Source: CAD feature listing. Evaluate the final solid. Frame: model axes, mm. Face numbers are marked on the shaded views. A direction names the side the tool comes from. Round coordinates to 2 decimals unless told otherwise and drop trailing zeros. Loops run counter-clockwise (first coordinate to the right, second up) from the corner with the lowest first, then second, coordinate; pieces in that order, holes last. Notation, with made-up numbers: M 22,9.25 L 43,9.25 A20 cw 43,25.25 Z; hole C 13,1.25 d11. An arc over 180 degrees is marked long. Write each question's results on one line, items separated by ' | '. Start each with the question number.
1. Section D-D on z = 10. Output: boundary loops of the cut face in (x, y), and give its area (3 significant figures).
2. Draft query along Z for the marked faces 6, 7 and 8. Return one class per face: released by +Z, released by -Z, zero draft, split by the parting line, or undercut.
3. Contact query for flat-ended pins moving along their axis: pin 1 Ø8 at (y, z) = (45.5, 0.5) entering from -X; pin 2 Ø3 at (x, z) = (-0.5, -10.5) entering from +Y; pin 3 Ø12 at (x, z) = (-13, -4.5) entering from +Y. Output: stop coordinate, or through.
4. Section A-A on x = 0. Output: boundary loops of the cut face in (y, z) (3 decimals), and give its area (3 significant figures).
5. Section C-C on y = 52. Output: boundary loops of the cut face in (x, z).
6. Ray query, line 1 (X direction, y = 50, z = -6); line 2 (X direction, y = 32.5, z = 0.5); line 3 (Y direction, x = -9.5, z = -3). Return the intervals inside material, ascending.
7. Set-up query: the marked faces 1, 2, 3, 4 and 5. Return all of +Z, -Z, +X, -X, +Y, -Y with unobstructed straight access to the full face (end or side cutting, diameter ignored); none if empty.
8. Section B-B on z = 1. Output: boundary loops of the cut face in (x, y).
from build123d import *

# Parameters (mm, degrees)
SKETCH1_R               = 12.9921
BOSS_EXTRUDE1_DEPTH     = 25.4
CUT_EXTRUDE1_DEPTH      = 71.405666164
CUT_EXTRUDE1_DEPTH_BACK = 71.405666164
SKETCH3_R               = 3.81
CUT_REVOLVE1_ANGLE      = 270
CUT_REVOLVE2_ANGLE      = 270
SKETCH6_R               = 8.255
CUT_EXTRUDE2_DEPTH      = 2.032
CUT_EXTRUDE3_DEPTH      = 24.638


with BuildPart() as part:
    # Sketch1 → Boss-Extrude1 (new body)
    with BuildSketch(Plane(origin=(0, 0, 0), x_dir=(1, 0, 0), z_dir=(0, 1, 0))):
        with Locations(Location((0, 0, 0), (0, 0, 270))):
            Circle(SKETCH1_R)
    extrude(amount=BOSS_EXTRUDE1_DEPTH)

    # Sketch2 → Revolve1 (revolve)
    with BuildSketch(Plane(origin=(0, 0, 0), x_dir=(0, 0, -1), z_dir=(1, 0, 0))):
        with BuildLine():
            Line((-16.764, 25.4), (-16.764, 49.53))
            ThreePointArc((-16.764, 49.53), (-11.85393808, 61.38393808), (0, 66.294))
            Line((0, 66.294), (0, 25.4))
            Line((0, 25.4), (-16.764, 25.4))
        make_face()
    revolve(axis=Axis((0, 25.4, 0), (0, 1, 0)))

    # Sketch3 → Cut-Extrude1 (cut, two sides: drawn at the far end of the back side and taken through both)
    with BuildSketch(Plane(origin=(0, 0, 0), x_dir=(0, 0, -1), z_dir=(1, 0, 0)).offset(-CUT_EXTRUDE1_DEPTH_BACK)):
        with Locations((0, 49.53)):
            Circle(SKETCH3_R)
    extrude(amount=CUT_EXTRUDE1_DEPTH + CUT_EXTRUDE1_DEPTH_BACK, mode=Mode.SUBTRACT)

    # Sketch4 → Cut-Revolve1 (revolve, cut)
    with BuildSketch(Plane.XY):
        with BuildLine():
            Line((-7.62, 32.995439638), (-7.62, 49.53))
            Line((-7.62, 49.53), (7.62, 49.53))
            Line((7.62, 49.53), (7.62, 32.995439638))
            ThreePointArc((7.62, 32.995439638), (0, 31.32406453), (-7.62, 32.995439638))
        make_face()
    revolve(axis=Axis((-7.62, 49.53, 0), (1, 0, 0)), revolution_arc=CUT_REVOLVE1_ANGLE, mode=Mode.SUBTRACT)

    # Sketch5 → Cut-Revolve2 (revolve, cut)
    with BuildSketch(Plane.XY):
        with BuildLine():
            Line((7.62, 53.34), (-7.62, 53.34))
            Line((-7.62, 53.34), (-7.62, 36.575518946))
            ThreePointArc((-7.62, 36.575518946), (0, 34.925), (7.62, 36.575518946))
            Line((7.62, 36.575518946), (7.62, 53.34))
        make_face()
    revolve(axis=Axis((7.62, 53.34, 0), (-1, 0, 0)), revolution_arc=CUT_REVOLVE2_ANGLE, mode=Mode.SUBTRACT)

    # Sketch6 → Cut-Extrude2 (cut)
    with BuildSketch(Plane(origin=(16.764, 0, 0), x_dir=(0, 0, -1), z_dir=(1, 0, 0))):
        with Locations((0, 49.53)):
            Circle(SKETCH6_R)
    cut_extrude2 = extrude(amount=-CUT_EXTRUDE2_DEPTH, mode=Mode.SUBTRACT)

    # Mirror1: Cut-Extrude2 across plane
    add(cut_extrude2.mirror(Plane(origin=(0, 0, 0), x_dir=(0, 0, 1), z_dir=(1, 0, 0))), mode=Mode.SUBTRACT)

    # Sketch7 → Cut-Extrude3 (cut)
    with BuildSketch(Plane.XY):
        with BuildLine():
            Line((-7.62, 49.53), (-7.62, 42.063955264))
            ThreePointArc((-7.62, 42.063955264), (0, 38.862), (7.62, 42.063955264))
            Line((7.62, 42.063955264), (7.62, 49.53))
            Line((7.62, 49.53), (-7.62, 49.53))
        make_face()
    extrude(amount=CUT_EXTRUDE3_DEPTH, mode=Mode.SUBTRACT)


solid = part.part
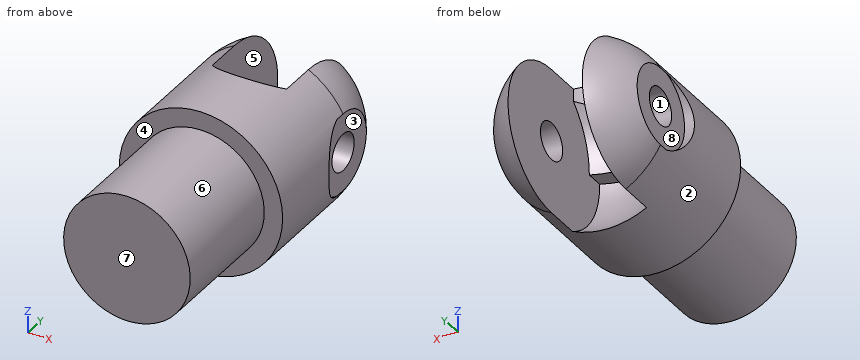
Taken from the geometry:
1) outline: M -13.45,25.4 L -8.29,25.4 L -8.29,0 L 8.29,0 L 8.29,25.4 L 13.45,25.4 L 13.45,49.53 A13.45 ccw 7.62,60.62 L 7.62,39.88 A15.46 cw -7.62,39.88 L -7.62,60.62 A13.45 ccw -13.45,49.53 Z | area: 994 mm^2
2) face 6: split by the parting line | face 7: zero draft | face 8: undercut
3) pin 1: x = -14.73 | pin 2: y = 35.85 | pin 3: y = 64.35
4) outline: M 0,-12.992 L 25.4,-12.992 L 25.4,-16.764 L 42.429,-16.764 A18.206 cw 31.324,0 L 34.925,0 A18.415 cw 38.862,11.38 L 38.862,16.764 L 25.4,16.764 L 25.4,12.992 L 0,12.992 Z | area: 1,010 mm^2
5) outline: M -14.73,-7.61 A16.58 ccw -7.62,-14.73 L -7.62,-2.9 L -14.73,-2.9 Z; M -14.73,2.9 L -7.62,2.9 L -7.62,14.73 A16.58 ccw -14.73,7.61 Z; M 7.62,-14.73 A16.58 ccw 14.73,-7.61 L 14.73,-2.9 L 7.62,-2.9 Z; M 7.62,2.9 L 14.73,2.9 L 14.73,7.61 A16.58 ccw 7.62,14.73 Z
6) line 1: -14.73 to -7.62, 7.62 to 14.73 | line 2: -16.76 to 16.76 | line 3: 0 to 47.18, 51.88 to 63.01
7) face 1: +X, -X | face 2: +Y, -Y | face 3: +X, +Y | face 4: -Y | face 5: +Y
8) outline: M -16.73,25.4 L -12.95,25.4 L -12.95,0 L 12.95,0 L 12.95,25.4 L 16.73,25.4 L 16.73,41.34 L 14.73,41.34 L 14.73,45.85 L 7.62,45.85 L 7.62,36.61 A18.39 cw -7.62,36.61 L -7.62,45.85 L -14.73,45.85 L -14.73,41.34 L -16.73,41.34 Z; M -14.73,53.21 L -7.62,53.21 L -7.62,64.43 A16.73 ccw -14.73,57.47 Z; M 7.62,53.21 L 14.73,53.21 L 14.73,57.47 A16.73 ccw 7.62,64.43 Z
